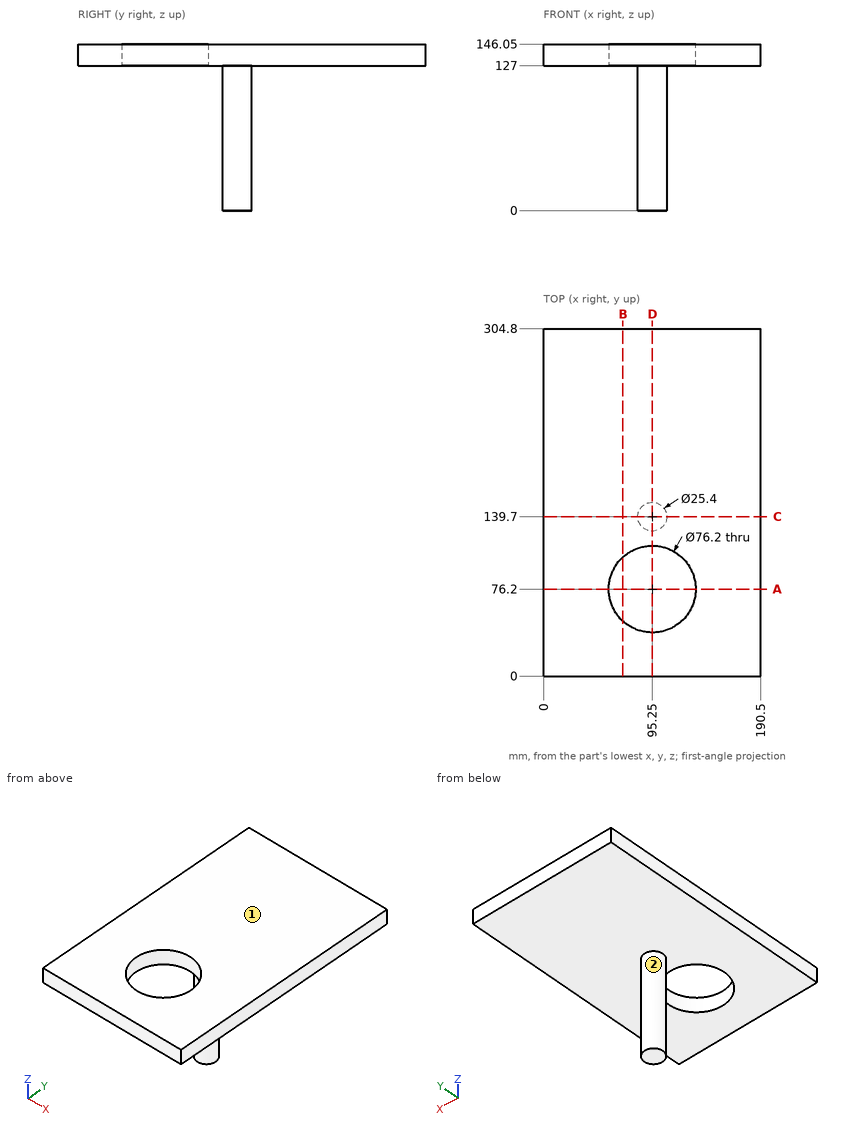
Check sheet for the drawn part. Datum: minimum x, y, z corner. Units: mm. A direction names the side the tool comes from. Round coordinates to 2 decimals unless told otherwise and drop trailing zeros. Order: outer loops, then holes, each group sorted by start corner. A loop starts at its lowest first (then second) coordinate and runs counter-clockwise, first axis right, second up.
1) Section check C-C (y = 139.7). Record the boundary of the cut face in (x, z), and give its area (3 significant figures).
2) Go/stop test with flat-tipped pins: pin 1 Ø8 at (x, y) = (82.5, 204.5) entering from -Z; pin 2 Ø1 at (x, z) = (105, 52) entering from -Y. Record where each tip stops, or that it passes through.
3) Section check B-B (x = 69.5). Record the boundary of the cut face in (y, z).
4) Tool access check on the marked faces 1 and 2. Record the directions out of +Z, -Z, +X, -X, +Y, -Y that give a thin tool (end or side, any length) a straight path to the whole face; none if there is none.
5) Scan lines: line 1 (X direction, y = 76, z = 141); line 2 (Y direction, x = 95.25, z = 138); line 3 (Z direction, x = 65, y = 184). Record each from-to range of solid material in increasing order.
6) Section check A-A (y = 76.2). Record the boundary of the cut face in (x, z).
7) Section check D-D (x = 95.25). Record the boundary of the cut face in (y, z).
Result:
1. outline: (0, 127) - (82.55, 127) - (82.55, 0) - (107.95, 0) - (107.95, 127) - (190.5, 127) - (190.5, 146.05) - (0, 146.05) - close
1. area: 6,850 mm2
2. pin 1: stops at z = 127
2. pin 2: stops at y = 131
3. outline: (0, 127) - (48.12, 127) - (48.12, 146.05) - (0, 146.05) - close; (104.28, 127) - (304.8, 127) - (304.8, 146.05) - (104.28, 146.05) - close
4. face 1: +Z, +X, -X, +Y, -Y
4. face 2: -Z
5. line 1: x = 0 to 57.15, 133.35 to 190.5
5. line 2: y = 0 to 38.1, 114.3 to 304.8
5. line 3: z = 127 to 146.05
6. outline: (0, 127) - (57.15, 127) - (57.15, 146.05) - (0, 146.05) - close; (133.35, 127) - (190.5, 127) - (190.5, 146.05) - (133.35, 146.05) - close
7. outline: (0, 127) - (38.1, 127) - (38.1, 146.05) - (0, 146.05) - close; (114.3, 127) - (127, 127) - (127, 0) - (152.4, 0) - (152.4, 127) - (304.8, 127) - (304.8, 146.05) - (114.3, 146.05) - close
